from build123d import *

# Parameters (mm, degrees)
F0_R     = 4
F1_DEPTH = 4


with BuildPart() as f1:
    # F0 (on Top) → F1 (new body)
    with BuildSketch(Plane.XY):
        with BuildLine():
            Line((2.5, -35), (11.9675303731, -3.6094621162))
            ThreePointArc((11.9675303731, -3.6094621162), (0, 12.5), (-11.9675303731, -3.6094621162))
            Line((-11.9675303731, -3.6094621162), (-2.5, -35))
            Line((-2.5, -35), (2.5, -35))
        make_face()
        Circle(F0_R, mode=Mode.SUBTRACT)
    extrude(amount=F1_DEPTH)

    # F4: sweep along a path in F4_path
    with BuildLine(Plane(origin=(-11.9675303731, -3.6094621162, 4), x_dir=(0, 1, 0), z_dir=(0, 0, 1))) as f4_path:
        Line((-31.3905378838, -9.4675303731), (0, 0))
        ThreePointArc((0, 0), (16.1094621162, -11.9675303731), (0, -23.9350607463))
        Line((0, -23.9350607463), (-31.3905378838, -14.4675303731))
        Line((-31.3905378838, -14.4675303731), (-38.5466098599, -12.309226204))
    # F3 (on face) → F4 (sweep, cut)
    with BuildSketch(Plane.XZ.offset(35)):
        with BuildLine():
            ThreePointArc((-2.5, 0.5358983849), (-1.0358983849, 2), (-0.5, 4))
            Line((-0.5, 4), (-2.5, 4))
            Line((-2.5, 4), (-2.5, 0.5358983849))
        make_face()
    sweep(path=f4_path.line, mode=Mode.SUBTRACT)

    # F5: F1 across face


with BuildPart() as f1_1:
    add(f1.part)
    add(f1.part.mirror(Plane(origin=(-0.0002320259, -7.7910771971, 4), x_dir=(1, 0, 0), z_dir=(0, 0, 1))))


solid = f1_1.part
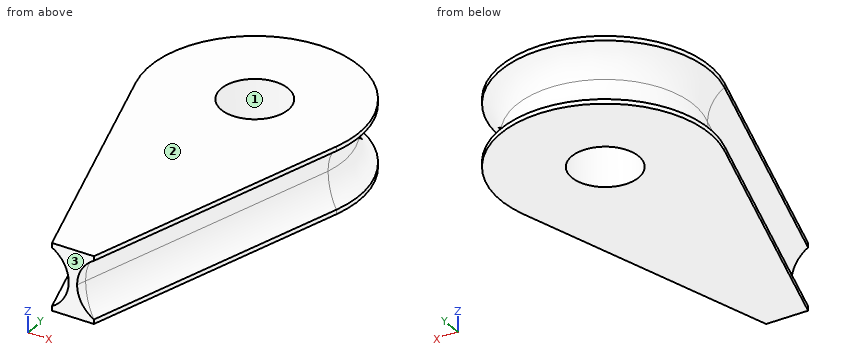
Check sheet for the modelled part. Datum: model origin and axes. Units: mm. Face numbers are marked on the shaded views. Round coordinates to 2 decimals unless told otherwise and drop trailing zeros.
(1) Go/stop test with flat-tipped pins: P1, Ø2, axis at y = 0, z = 6, coming from the +X side; P2, Ø3, axis at x = -8, y = -8.5, coming from the -Z side; P3, Ø1, axis at x = 2, z = 3.5, coming from the +Y side. Record where each tip stops, or that it passes through.
(2) Scan lines: probe 1 along X at (y, z) = (1, 7.5); probe 2 along Y at (x, z) = (0, 4.25); probe 3 along X at (y, z) = (-30, 2). Record each from-to range of solid material in increasing order.
(3) Draft check along Y on the marked faces 1, 2 and 3. Enter one of: pulls with the +Y half, pulls with the -Y half, needs draft (parallel to the pull), parting line crosses it, or undercut.
Check sheet entries:
1. P1: stops at x = 11.88
1. P2: stops at z = 0
1. P3: stops at y = 10.56
2. probe 1: x = -12.46 to -3.87, 3.87 to 12.46
2. probe 2: y = -35 to -4, 4 to 10.61
2. probe 3: x = -2.54 to 2.54
3. face 1: undercut
3. face 2: needs draft
3. face 3: pulls with the -Y half
